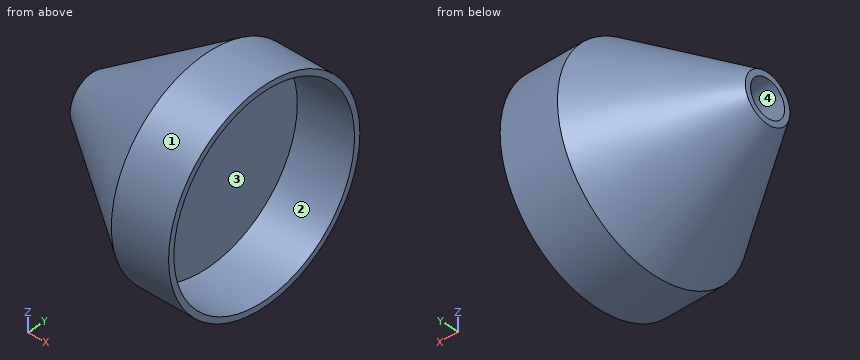
```python
from build123d import *

# Parameters (mm, degrees)
F0_R     = 2.1
F2_R     = 9
F4_R     = 1.6
F5_DEPTH = 5
F6_DEPTH = 5
F7_R     = 8.5
F8_DEPTH = 5


with BuildPart() as f3:
    # F0 (on Right) → F3 section 0
    with BuildSketch(Plane.YZ):
        Circle(F0_R)
    # F2 (on offset) → F3 section 1
    with BuildSketch(Plane.YZ.offset(10)):
        Circle(F2_R)
    loft()

    # F4 (on face) → F5 (cut)
    with BuildSketch(Plane(origin=(0, 0, 0), x_dir=(0, -1, 0), z_dir=(-1, 0, 0))):
        Circle(F4_R)
    extrude(amount=-F5_DEPTH, mode=Mode.SUBTRACT)

    # F2 (on offset) → F6 (join)
    with BuildSketch(Plane.YZ.offset(10)):
        Circle(F2_R)
    extrude(amount=F6_DEPTH)

    # F7 (on face) → F8 (cut)
    with BuildSketch(Plane.YZ.offset(15)):
        Circle(F7_R)
    extrude(amount=-F8_DEPTH, mode=Mode.SUBTRACT)


solid = f3.part
```
CAD build for the part. Positions are in the model's coordinates, mm. Face numbers are marked on the shaded views. A direction names the side the tool comes from. Coordinates: 2 decimals unless noted, no trailing zeros. Write each loop counter-clockwise with the first axis right and the second up, starting at its lowest first coordinate (ties: lowest second). Pieces come first, ordered by that corner, then holes. Notation, with made-up numbers: (-38, 18) -> (-30, 18) arc R15 cw to (-30, 38) -> close; hole circle Ø4 at (68.25, 49.5). An arc over 180 degrees is marked (long way). Return JSON: item names as keys, results as strings. Group by question number.
Q1. Pull direction Z, two halves, no side cores. Call the marked faces 1 and 2: released by +Z, released by -Z, zero draft, split by the parting line, or undercut.
Q2. Cut at C-C, the plane x = 1. Give the cut face in (y, z), then the cut area to 3 significant figures.
Q3. Cut at D-D, the plane x = 9.75. Give the cut face in (y, z) (1 decimal).
Q4. Which spindle directions (+Z, -Z, +X, -X, +Y, -Y) get a long thin tool onto all of the face, cutting with end or side? Do the marked faces 3 and 4. Say none if no direction does.
Q5. Drill centre lines: line 1 (Z direction, x = 12.2, y = 0); line 2 (Z direction, x = 2.9, y = 0); line 3 (Y direction, x = 2.25, z = 1). Where is each one in solid material? Low to high.
Q6. Flat gauge pins, fed straight in: pin 1 (4 mm diameter, centred on x = 4, z = 1, fed in from -Y); pin 2 (1.5 mm diameter, centred on y = -3, z = -1.5, fed in from +X); pin 3 (1.6 mm diameter, centred on y = 0, z = -0.5, fed in from -X). Where does each tip first touch, or does it go through?
Q7. Cut at B-B, the plane x = 3. Give the cut face in (y, z).
Q8. Cut at A-A, the plane y = 0. Give the cut face in (x, z), then the cut area to 4 significant figures.
Returned:
{
 "1": {"face 1": "split by the parting line", "face 2": "undercut"},
 "2": {"outline": "circle Ø5.58 at (0, 0); hole circle Ø3.2 at (0, 0)", "area": "16.4 mm2"},
 "3": {"outline": "circle Ø17.7 at (0, 0)"},
 "4": {"face 3": "+X", "face 4": "-X"},
 "5": {"line 1": "z = -9 to -8.5, 8.5 to 9", "line 2": "z = -4.1 to -1.6, 1.6 to 4.1", "line 3": "y = -3.51 to -1.25, 1.25 to 3.51"},
 "6": {"pin 1": "stops at y = -6.18", "pin 2": "stops at x = 10", "pin 3": "stops at x = 5"},
 "7": {"outline": "circle Ø8.34 at (0, 0); hole circle Ø3.2 at (0, 0)"},
 "8": {"outline": "(0, -2.1) -> (10, -9) -> (15, -9) -> (15, -8.5) -> (10, -8.5) -> (10, 8.5) -> (15, 8.5) -> (15, 9) -> (10, 9) -> (0, 2.1) -> (0, 1.6) -> (5, 1.6) -> (5, -1.6) -> (0, -1.6) -> close", "area": "100.0 mm2"}
}
